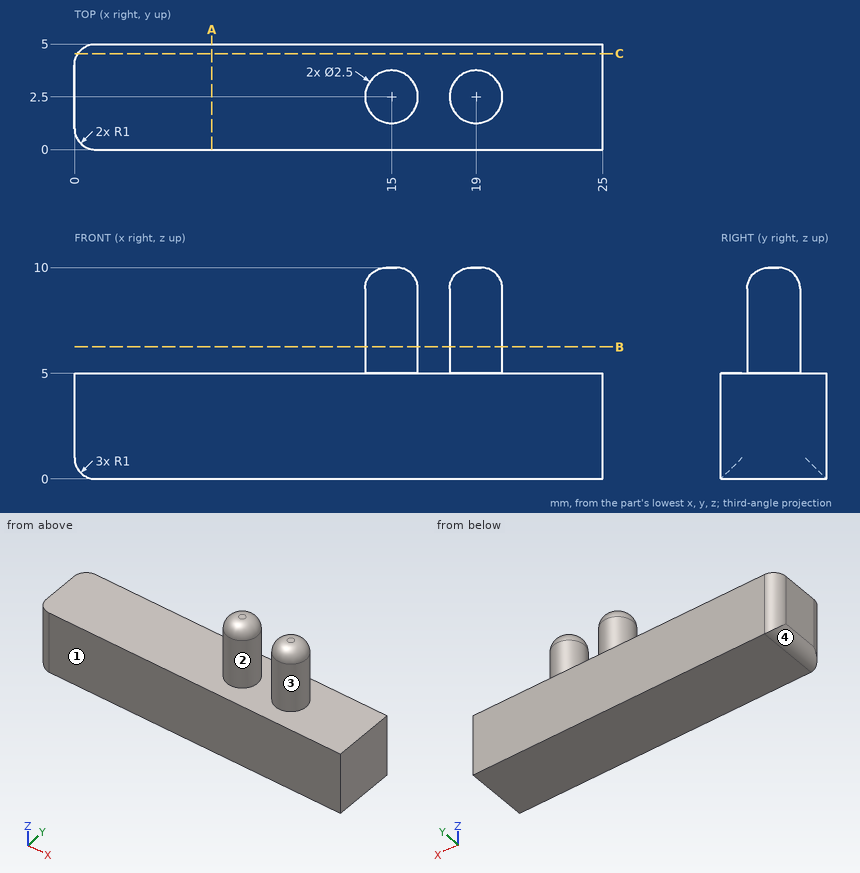
Check sheet for the drawn part. Datum: minimum x, y, z corner. Units: mm. Round coordinates to 2 decimals unless told otherwise and drop trailing zeros. Loops run counter-clockwise (first coordinate to the right, second up) from the corner with the lowest first, then second, coordinate; pieces in that order, holes last. Notation, with made-up numbers: (49.25, 30) -> (106.25, 30) arc R22 cw to (106.25, 49) -> close; hole circle Ø6 at (-40, 33.5). An arc over 180 degrees is marked (long way). Put each result on its own line as item: value. Start each with the question number.
1. Draft check along X on the marked faces 1, 2, 3 and 4. Enter one of: +X half, -X half, draft (parallel to the pull), parting line (faces both ways), or undercut.
2. Section check B-B (z = 6.25). Enter the section's corners in (x, y), plus the area to 3 significant figures.
3. Section check A-A (x = 6.5). Enter the section's corners in (y, z), plus the area to 3 significant figures.
4. Scan lines: probe 1 along Z at (x, y) = (9.5, 1.05); probe 2 along X at (y, z) = (1.55, 8.25); probe 3 along X at (y, z) = (2.8, 7.25). Record each from-to range of solid material in increasing order.
5. Gauge pin test, flat ends, axial feed: pin 1 (1 mm diameter, centred on y = 3, z = 9, fed in from +X); pin 2 (2 mm diameter, centred on x = 10, z = 6.5, fed in from +Y). Record the tip position at first contact, or that the pin passes through.
6. Section check C-C (y = 4.55). Enter the section's corners in (x, z).
Findings:
1. face 1: draft
1. face 2: undercut
1. face 3: undercut
1. face 4: -X half
2. outline: circle Ø2.5 at (15, 2.5); circle Ø2.5 at (19, 2.5)
2. area: 9.82 mm^2
3. outline: (0, 0) -> (5, 0) -> (5, 5) -> (0, 5) -> close
3. area: 25.0 mm^2
4. probe 1: z = 0 to 5
4. probe 2: x = 14.19 to 15.81, 18.19 to 19.81
4. probe 3: x = 13.79 to 16.21, 17.79 to 20.21
5. pin 1: stops at x = 20.25
5. pin 2: passes through
6. outline: (0.16, 0.45) arc R1 ccw to (1, 0) -> (25, 0) -> (25, 5) -> (0.16, 5) -> close
